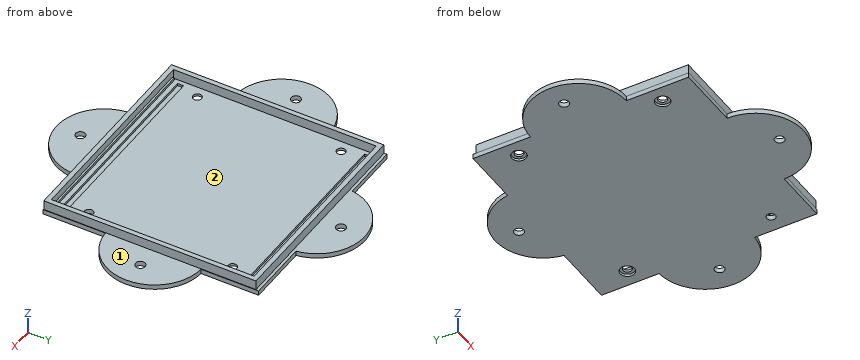
from build123d import *

# Parameters (mm, degrees)
CYLINDER015_R          = 1.8
CYLINDER015_DEPTH      = 300
CYLINDER013_R          = 1.8
CYLINDER013_DEPTH      = 300
CYLINDER012_R          = 1.8
CYLINDER012_DEPTH      = 300
BOX034_W               = 82
BOX034_H               = 2.5
BOX034_DEPTH           = 1
BOX030_W               = 82
BOX030_H               = 2.5
BOX030_DEPTH           = 1
CYLINDER016_R          = 3
CYLINDER016_DEPTH      = 1
CYLINDER017_R          = 3
CYLINDER017_DEPTH      = 1
CYLINDER018_R          = 3
CYLINDER018_DEPTH      = 1
CYLINDER014_R          = 1.8
CYLINDER014_DEPTH      = 300
BOX035_W               = 84
BOX035_H               = 2
BOX035_DEPTH           = 2
BOX038_W               = 85.6
BOX038_H               = 84.6
BOX038_DEPTH           = 4
THICKNESS001_T         = 2
CYLINDER022_R          = 2
CYLINDER022_DEPTH      = 10
CYLINDER021_R          = 20
CYLINDER021_DEPTH      = 2
CYLINDER023_R          = 2
CYLINDER023_DEPTH      = 10
CYLINDER020_R          = 20
CYLINDER020_DEPTH      = 2
CYLINDER026_R          = 2
CYLINDER026_DEPTH      = 10
CYLINDER027_W          = 20
CYLINDER027_H          = 2
CYLINDER027_ANGLE      = 180
CUT007_PLACEMENT_ANGLE = 90
CYLINDER024_R          = 2
CYLINDER024_DEPTH      = 10
CYLINDER025_W          = 20
CYLINDER025_H          = 2
CYLINDER025_ANGLE      = 180
CUT006_PLACEMENT_ANGLE = 90
BOX029_W               = 90
BOX029_H               = 90
BOX029_DEPTH           = 2


with BuildPart() as cylinder015:
    # Cylinder015 → Cylinder015 (new body)
    with BuildSketch(Plane(origin=(2, 70, -69), x_dir=(1, 0, 0), z_dir=(0, 0, 1))):
        Circle(CYLINDER015_R)
    extrude(amount=CYLINDER015_DEPTH)


with BuildPart() as cylinder013:
    # Cylinder013 → Cylinder013 (new body)
    with BuildSketch(Plane(origin=(78, 70, -107), x_dir=(1, 0, 0), z_dir=(0, 0, 1))):
        Circle(CYLINDER013_R)
    extrude(amount=CYLINDER013_DEPTH)


with BuildPart() as cylinder012:
    # Cylinder012 → Cylinder012 (new body)
    with BuildSketch(Plane(origin=(78, 10, -70), x_dir=(1, 0, 0), z_dir=(0, 0, 1))):
        Circle(CYLINDER012_R)
    extrude(amount=CYLINDER012_DEPTH)


with BuildPart() as cube022:
    # Box034 → Box034 (new body)
    with BuildSketch(Plane(origin=(-1, 78, 1), x_dir=(1, 0, 0), z_dir=(0, 0, 1))):
        with Locations((41, 1.25)):
            Rectangle(BOX034_W, BOX034_H)
    extrude(amount=BOX034_DEPTH)


with BuildPart() as cube018:
    # Box030 → Box030 (new body)
    with BuildSketch(Plane(origin=(-1, 0, 1), x_dir=(1, 0, 0), z_dir=(0, 0, 1))):
        with Locations((41, 1.25)):
            Rectangle(BOX030_W, BOX030_H)
    extrude(amount=BOX030_DEPTH)


with BuildPart() as cylinder016:
    # Cylinder016 → Cylinder016 (new body)
    with BuildSketch(Plane(origin=(2, 10, 0), x_dir=(1, 0, 0), z_dir=(0, 0, 1))):
        Circle(CYLINDER016_R)
    extrude(amount=CYLINDER016_DEPTH)


with BuildPart() as cylinder017:
    # Cylinder017 → Cylinder017 (new body)
    with BuildSketch(Plane(origin=(2, 70, 0), x_dir=(1, 0, 0), z_dir=(0, 0, 1))):
        Circle(CYLINDER017_R)
    extrude(amount=CYLINDER017_DEPTH)


with BuildPart() as cylinder018:
    # Cylinder018 → Cylinder018 (new body)
    with BuildSketch(Plane(origin=(78, 70, 0), x_dir=(1, 0, 0), z_dir=(0, 0, 1))):
        Circle(CYLINDER018_R)
    extrude(amount=CYLINDER018_DEPTH)


with BuildPart() as fusion008:
    # Cylinder014 → Cylinder014 (new body)
    with BuildSketch(Plane(origin=(2, 10, -63), x_dir=(1, 0, 0), z_dir=(0, 0, 1))):
        Circle(CYLINDER014_R)
    extrude(amount=CYLINDER014_DEPTH)

    # Fusion008: union Cylinder015, Cylinder013, Cylinder012, Cube022, Cube018, Cylinder016, Cylinder017, Cylinder018
    add(cylinder015.part)
    add(cylinder013.part)
    add(cylinder012.part)
    add(cube022.part)
    add(cube018.part)
    add(cylinder016.part)
    add(cylinder017.part)
    add(cylinder018.part)


with BuildPart() as cube023:
    # Box035 → Box035 (new body)
    with BuildSketch(Plane(origin=(-2, -4, 1), x_dir=(1, 0, 0), z_dir=(0, 0, 1))):
        with Locations((42, 1)):
            Rectangle(BOX035_W, BOX035_H)
    extrude(amount=BOX035_DEPTH)


with BuildPart() as thickness001:
    # Box038 → Box038 (new body)
    with BuildSketch(Plane(origin=(-2.8, -2.8, 2), x_dir=(1, 0, 0), z_dir=(0, 0, 1))):
        with Locations((42.8, 42.3)):
            Rectangle(BOX038_W, BOX038_H)
    extrude(amount=BOX038_DEPTH)

    # Thickness001
    thickness001_openings = [thickness001.faces().sort_by_distance(p)[0] for p in [
        (40, 39.5, 2),
        (40, 39.5, 6),
    ]]
    offset(amount=THICKNESS001_T, openings=thickness001_openings, kind=Kind.INTERSECTION)


with BuildPart() as cylinder022:
    # Cylinder022 → Cylinder022 (new body)
    with BuildSketch(Plane(origin=(94, 41, 0), x_dir=(1, 0, 0), z_dir=(0, 0, 1))):
        Circle(CYLINDER022_R)
    extrude(amount=CYLINDER022_DEPTH)


with BuildPart() as cut004:
    # Cylinder021 → Cylinder021 (new body)
    with BuildSketch(Plane(origin=(84, 41, 0), x_dir=(1, 0, 0), z_dir=(0, 0, 1))):
        Circle(CYLINDER021_R)
    extrude(amount=CYLINDER021_DEPTH)

    # Cut004: cut Cylinder022
    add(cylinder022.part, mode=Mode.SUBTRACT)


with BuildPart() as cylinder023:
    # Cylinder023 → Cylinder023 (new body)
    with BuildSketch(Plane(origin=(-15, 41, 0), x_dir=(1, 0, 0), z_dir=(0, 0, 1))):
        Circle(CYLINDER023_R)
    extrude(amount=CYLINDER023_DEPTH)


with BuildPart() as cut005:
    # Cylinder020 → Cylinder020 (new body)
    with BuildSketch(Plane(origin=(-5, 41, 0), x_dir=(1, 0, 0), z_dir=(0, 0, 1))):
        Circle(CYLINDER020_R)
    extrude(amount=CYLINDER020_DEPTH)

    # Cut005: cut Cylinder023
    add(cylinder023.part, mode=Mode.SUBTRACT)


with BuildPart() as cylinder026:
    # Cylinder026 → Cylinder026 (new body)
    with BuildSketch(Plane(origin=(-15, 41, 0), x_dir=(1, 0, 0), z_dir=(0, 0, 1))):
        Circle(CYLINDER026_R)
    extrude(amount=CYLINDER026_DEPTH)


with BuildPart() as cut007:
    # Cylinder027 → Cylinder027 (revolve)
    with BuildSketch(Plane(origin=(-5, 41, 0), x_dir=(0, 1, 0), z_dir=(1, 0, 0))):
        with Locations((10, 1)):
            Rectangle(CYLINDER027_W, CYLINDER027_H)
    revolve(axis=Axis((-5, 41, 0), (0, 0, 1)), revolution_arc=CYLINDER027_ANGLE)

    # Cut007: cut Cylinder026
    add(cylinder026.part, mode=Mode.SUBTRACT)


with BuildPart() as cut007_1:
    # Cut007 placement: moved
    add(cut007.part.moved(Location((-2, 77, 0))).rotate(Axis((-2, 77, 0), (0, 0, -1)), CUT007_PLACEMENT_ANGLE))


with BuildPart() as cylinder024:
    # Cylinder024 → Cylinder024 (new body)
    with BuildSketch(Plane(origin=(-15, 41, 0), x_dir=(1, 0, 0), z_dir=(0, 0, 1))):
        Circle(CYLINDER024_R)
    extrude(amount=CYLINDER024_DEPTH)


with BuildPart() as cut006:
    # Cylinder025 → Cylinder025 (revolve)
    with BuildSketch(Plane(origin=(-5, 41, 0), x_dir=(0, 1, 0), z_dir=(1, 0, 0))):
        with Locations((10, 1)):
            Rectangle(CYLINDER025_W, CYLINDER025_H)
    revolve(axis=Axis((-5, 41, 0), (0, 0, 1)), revolution_arc=CYLINDER025_ANGLE)

    # Cut006: cut Cylinder024
    add(cylinder024.part, mode=Mode.SUBTRACT)


with BuildPart() as cut006_1:
    # Cut006 placement: moved
    add(cut006.part.moved(Location((83, 0, 0))).rotate(Axis((83, 0, 0), (0, 0, 1)), CUT006_PLACEMENT_ANGLE))


with BuildPart() as obj1:
    # Box029 → Box029 (new body)
    with BuildSketch(Plane(origin=(-5, -5, 0), x_dir=(1, 0, 0), z_dir=(0, 0, 1))):
        with Locations((45, 45)):
            Rectangle(BOX029_W, BOX029_H)
    extrude(amount=BOX029_DEPTH)

    # Fusion007: union Cube023, Thickness001, Cut004, Cut005, Cut007, Cut006
    add(cube023.part)
    add(thickness001.part)
    add(cut004.part)
    add(cut005.part)
    add(cut007_1.part)
    add(cut006_1.part)

    # Cut003: cut Fusion008
    add(fusion008.part, mode=Mode.SUBTRACT)


solid = obj1.part
Design review of the part built by this model. Coordinates are the model's own, in mm. Face numbers are marked on the shaded views. Coordinates: 2 decimals unless noted, no trailing zeros. Loops run counter-clockwise (first coordinate to the right, second up) from the corner with the lowest first, then second, coordinate; pieces in that order, holes last. Notation, with made-up numbers: (-5, -23) - (14, -23) arc R35 ccw to (14, 16) - close; hole circle Ø9 at (72, 82.5). An arc over 180 degrees is marked (long way). Use CSV: the item, a comma, the result in double quotes. Start each with the question number.
1. Add section D-D on x = 67.5. Give the boundary of the cut face in (y, z).
2. Add section C-C on x = 94. Give the boundary of the cut face in (y, z), plus the area to 3 significant figures.
3. Add section A-A on z = 5. Give the boundary of the cut face in (x, y), plus the area to 3 significant figures.
4. Clearance check with flat-ended pins moving along their axes: pin 1 (0.6 mm diameter, centred on x = 7.5, z = 1, fed in from +Y); pin 2 (4.5 mm diameter, centred on x = 42, y = -15, fed in from -Z); pin 3 (1.1 mm diameter, centred on x = 48.5, z = 1.5, fed in from -Y); pin 4 (3 mm diameter, centred on x = 78, y = 70, fed in from +Z). State where each tip first meets the part, or that it passes through.
5. Add section B-B on y = 92. Give the boundary of the cut face in (x, z), plus the area to 3 significant figures.
6. To check wall thickness, follow probe 1 along X at (y, z) = (70, 1.55); probe 2 along Y at (x, z) = (78, 0.95); probe 3 along Y at (x, z) = (10.5, 1.45). State the ranges of each line that lie inside material, in increasing order.
7. Mouldability with a two-part tool opening along Y and no side actions: class the marked faces 1 and 2 as released by +Y, released by -Y, zero draft, split by the parting line, or undercut.
Resolved:
1,outline,"(-5, 0) - (85, 0) - (85, 2) - (83.8, 2) - (83.8, 6) - (81.8, 6) - (81.8, 2) - (80.5, 2) - (80.5, 1) - (78, 1) - (78, 2) - (2.5, 2) - (2.5, 1) - (0, 1) - (0, 2) - (-2, 2) - (-2, 3) - (-2.8, 3) - (-2.8, 6) - (-4.8, 6) - (-4.8, 2) - (-5, 2) - close"
2,outline,"(23.68, 0) - (39, 0) - (39, 2) - (23.68, 2) - close; (43, 0) - (58.32, 0) - (58.32, 2) - (43, 2) - close"
2,area,"61.3 mm2"
3,outline,"(-4.8, -4.8) - (84.8, -4.8) - (84.8, 83.8) - (-4.8, 83.8) - close; hole (-2.8, -2.8) - (82.8, -2.8) - (82.8, 81.8) - (-2.8, 81.8) - close"
3,area,"697 mm2"
4,pin 1,"y = 85"
4,pin 2,"z = 0"
4,pin 3,"y = -24.09"
4,pin 4,"through"
5,outline,"(21.68, 0) - (37, 0) - (37, 2) - (21.68, 2) - close; (41, 0) - (56.32, 0) - (56.32, 2) - (41, 2) - close"
5,area,"61.3 mm2"
6,probe 1,"-5 to 0.2, 3.8 to 76.2, 79.8 to 85"
6,probe 2,"-5 to 8.2, 11.8 to 67, 73 to 85"
6,probe 3,"-5 to 0, 2.5 to 78, 80.5 to 85"
7,face 1,"zero draft"
7,face 2,"undercut"
